from build123d import *

# Parameters (mm, degrees)
SKETCH1_W           = 300
SKETCH1_H           = 300
BOSS_EXTRUDE1_DEPTH = 10
BOSS_EXTRUDE4_DEPTH = 20


with BuildPart() as part:
    # Sketch1 → Boss-Extrude1 (new body)
    with BuildSketch(Plane(origin=(0, 0, 0), x_dir=(1, 0, 0), z_dir=(0, 1, 0))):
        Rectangle(SKETCH1_W, SKETCH1_H)
    extrude(amount=BOSS_EXTRUDE1_DEPTH)

    # Sketch2 → Boss-Extrude4 (add)
    with BuildSketch(Plane(origin=(0, 10, 0), x_dir=(1, 0, 0), z_dir=(0, 1, 0))):
        Polygon((49.971374343, 108.306734699), (-9.273843692, 108.306734699), (-9.273843692, 65.302548914), (39.109683003, 65.302548914), (39.109683003, -42.978794556), (-14.169964592, -42.978794556), (-14.169964592, -112.952152785), (33.151642128, -112.952152785), (33.151642128, -67.566816692), (30.802124143, -67.566816692), (30.802124143, -109.346745837), (-10.423438765, -109.346745837), (-10.423438765, -74.73050528), (9.957336402, -74.73050528), (9.957336402, -72.613697765), (-10.423438765, -72.613697765), (-10.423438765, -46.978265259), (42.650315476, -46.978265259), (42.650315476, 65.302548914), (95.184908211, 65.302548914), (95.184908211, -63.123542137), (73.07070507, -63.123542137), (73.07070507, -101.668120527), (76.534473407, -101.668120527), (76.534473407, -66.320866756), (99.982757345, -66.320866756), (99.982757345, 150), (-102.935144351, 150), (-102.935144351, 77.901270739), (-43.092149345, 77.901270739), (-43.092149345, 80.20776174), (-100.595048935, 80.20776174), (-100.595048935, 105.650837757), (-37.989692586, 105.650837757), (-37.989692586, 108.306734699), (-100.595048935, 108.306734699), (-100.595048935, 147.003199663), (95.184908211, 147.003199663), (95.184908211, 68.375256183), (-6.232251129, 68.375256183), (-6.232251129, 105.650837757), (49.971374343, 105.650837757), (49.971374343, 94.342521139), (52.60088631, 94.342521139), (52.60088631, 124.362722745), (49.971374343, 124.362722745), align=None)
        Polygon((-146.001890411, 52.431305921), (-146.001890411, 150), (-150, 150), (-150, -150), (150, -150), (150, 150), (144.101294188, 150), (144.101294188, -91.584402299), (104.478721877, -91.584402299), (104.478721877, -119.965629386), (88.345614046, -119.965629386), (88.345614046, -145.94528604), (-114.452609493, -145.94528604), (-114.452609493, -47.69748233), (-83.008411836, -47.69748233), (-83.008411836, -20.290963527), (-86.710364357, -20.290963527), (-86.710364357, -43.614528655), (-118.021528945, -43.614528655), (-118.021528945, -111.174686517), (-145.802253378, -111.174686517), (-145.802253378, 49.940489366), (-58.285164429, 49.940489366), (-58.285164429, 33.250662457), (-92.45985442, 33.250662457), (-92.45985442, 30.093436444), (2.163221537, 30.093436444), (2.163221537, 12.78236321), (-95.832026153, 12.78236321), (-95.832026153, 9.764730819), (2.163221537, 9.764730819), (2.163221537, -11.779862869), (-55.377515494, -11.779862869), (-55.377515494, -114.277161571), (-83.335773751, -114.277161571), (-83.335773751, -83.046520825), (-86.246233134, -83.046520825), (-86.246233134, -117.269753185), (-51.991052188, -117.269753185), (-51.991052188, -15.009651935), (5.313331338, -15.009651935), (5.313331338, 33.250662457), (-55.651758488, 33.250662457), (-55.651758488, 52.431305921), align=None)
    extrude(amount=BOSS_EXTRUDE4_DEPTH)


solid = part.part
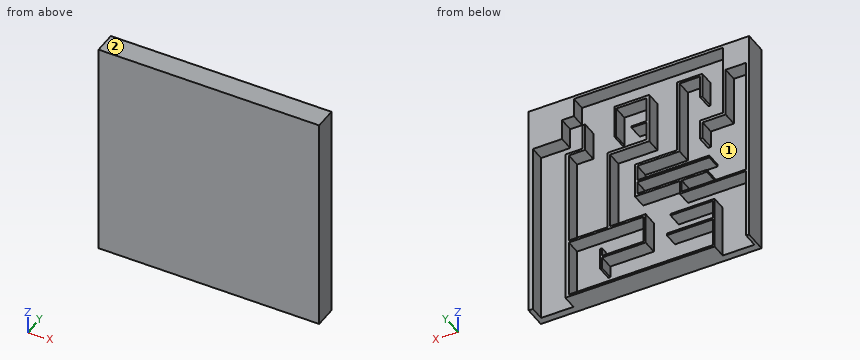
Source: CAD feature listing. Evaluate the final solid. Frame: model axes, mm. Face numbers are marked on the shaded views. Round coordinates to 2 decimals unless told otherwise and drop trailing zeros. Order: outer loops, then holes, each group sorted by start corner. A loop starts at its lowest first (then second) coordinate and runs counter-clockwise, first axis right, second up. Notation, with made-up numbers: (23, -29) - (41, -29) arc R13 ccw to (41, -14) - close; hole circle Ø2 at (52, 36). An arc over 180 degrees is marked (long way). Use a Markdown table: item, result. Add a question column.
1. Mould query, pull axis X, two halves, no side actions, for the marked faces 1 and 2. Classes: +X half, -X half, draft (parallel to the pull), parting line (faces both ways), or undercut.
2. Line query: probe 1 along X at (y, z) = (22, -37); probe 2 along X at (y, z) = (22.5, -74); probe 3 along Z at (x, y) = (32, 23). Output: solid intervals per line, ascending.
3. Section query A-A (x = -23). Return the cut outline in (y, z).
4. Section query B-B (z = 28). Return the cut outline in (x, y).
5. First-contact query: pin 1 (5 mm diameter, centred on x = -118, y = 27, fed in from -Z); pin 2 (5 mm diameter, centred on x = -107, z = -111, fed in from +Y). Flat tips, straight axial feed; report the tip coordinate or a pass-through.
6. Section query C-C (z = -39.5). Return the cut outline in (x, y).
Derived:
| question | item | result |
|---|---|---|
| 1 | face 1 | undercut |
| 1 | face 2 | draft |
| 2 | probe 1 | -150 to -145.8, -58.29 to -55.65, 39.11 to 42.65, 95.18 to 99.98, 144.1 to 150 |
| 2 | probe 2 | -150 to -146, -9.27 to -6.23, 95.18 to 99.98, 144.1 to 150 |
| 2 | probe 3 | -150 to -147, -108.31 to -105.65, -68.38 to -65.3, 42.98 to 46.98, 67.57 to 112.95, 145.95 to 150 |
| 3 | outline | (0, -150) - (30, -150) - (30, -147) - (10, -147) - (10, -33.25) - (30, -33.25) - (30, -30.09) - (10, -30.09) - (10, -12.78) - (30, -12.78) - (30, -9.76) - (10, -9.76) - (10, 11.78) - (30, 11.78) - (30, 15.01) - (10, 15.01) - (10, 145.95) - (30, 145.95) - (30, 150) - (0, 150) - close |
| 4 | outline | (-150, 0) - (150, 0) - (150, 30) - (144.1, 30) - (144.1, 10) - (99.98, 10) - (99.98, 30) - (95.18, 30) - (95.18, 10) - (42.65, 10) - (42.65, 30) - (39.11, 30) - (39.11, 10) - (-51.99, 10) - (-51.99, 30) - (-55.38, 30) - (-55.38, 10) - (-83.01, 10) - (-83.01, 30) - (-86.71, 30) - (-86.71, 10) - (-145.8, 10) - (-145.8, 30) - (-150, 30) - close |
| 5 | pin 1 | z = -52.43 |
| 5 | pin 2 | y = 10 |
| 6 | outline | (-150, 0) - (150, 0) - (150, 30) - (144.1, 30) - (144.1, 10) - (99.98, 10) - (99.98, 30) - (95.18, 30) - (95.18, 10) - (42.65, 10) - (42.65, 30) - (39.11, 30) - (39.11, 10) - (-55.65, 10) - (-55.65, 30) - (-58.29, 30) - (-58.29, 10) - (-145.8, 10) - (-145.8, 30) - (-150, 30) - close |
